Autodesk Inventor part; units mm, degrees
ref_plane "YZ Plane" through (0, 0, 0) normal (1, 0, 0) x (0, 1, 0)
ref_plane "XZ Plane" through (0, 0, 0) normal (0, 1, 0) x (-1, 0, 0)
ref_plane "XY Plane" through (0, 0, 0) normal (0, 0, 1) x (1, 0, 0)
sketch "Sketch1" plane through (0, 0, 0) normal (0, 1, 0) x (-1, 0, 0)
  line L0 (0, 0) -> (19.05, 0)
  line L1 (19.05, 0) -> (19.05, 44.45)
  line L2 (0, 19.05) -> (0, 0)
  circle A0 centre (9.525, 9.525) radius 6.35
  arc A1 (-166.7131, 44.45) -> (-166.7131, 19.05) centre (-215.9, 31.75) ccw
  line L3 (19.05, 44.45) -> (-41.3006, 44.45)
  line L4 (-139.6744, 44.45) -> (-166.7131, 44.45)
  line L5 (-166.7131, 19.05) -> (-139.6744, 19.05)
  line L6 (-41.3006, 19.05) -> (0, 19.05)
  arc A2 (-41.3006, 44.45) -> (-139.6744, 44.45) centre (-90.4875, 31.75) ccw
  arc A3 (-139.6744, 19.05) -> (-41.3006, 19.05) centre (-90.4875, 31.75) ccw
  dimension "d0" = 19.05
  dimension "d2" = 12.7
  dimension "d5" = 44.45
extrude "Extrusion1" add sketch "Sketch1" along normal blind 25.4
properties part number "wheels"
Read the model definition and answer for the solid it produces. Units are mm, in the model's axes. A direction names the side the tool comes from. Coordinates: 2 decimals unless noted, no trailing zeros. Write each loop counter-clockwise with the first axis right and the second up, starting at its lowest first coordinate (ties: lowest second). Pieces come first, ordered by that corner, then holes. Notation, with made-up numbers: (88, 59.5) - (136, 59.5) arc R15 cw to (136, 65.5) - close; hole circle Ø5 at (27, -32). An arc over 180 degrees is marked (long way). Answer as a JSON object with one key per item and string values. Group by question number.
1. A cutting plane is placed at D-D (z = 69.5). Determine the outline of the cut face in (x, y).
2. A cutting plane is placed at C-C (z = 13). Determine the outline of the cut face in (x, y), plus the area to 3 significant figures.
3. Which of the six approach directions +Z, -Z, +X, -X, +Y, -Y give full straight-line access (tool end or side, diameter ignored) to faces 1 (the flat face through (153, 13, 19.05)), 2 (the flat face through (153, 13, 44.45)), 3 (the flat face through (-9, 13, 0))?
4. Each of these flat-tipped pins is pushed along its axis until it touches: P1, Ø1.5, axis at y = 21, z = 69, coming from the +X side; P2, Ø15, axis at x = -7.5, y = 9.5, coming from the -Z side; P3, Ø1.5, axis at x = 86, y = 19.5, coming from the -Z side. Where does it stop, or does it pass through?
5. A cutting plane is placed at A-A (z = 52). Determine the outline of the cut face in (x, y).
6. The mould has two halves that part along X. Classify faces 4 (the flat face through (126, 25.4, 32)), 5 (the flat face through (-19.05, 13, 22)), 6 (the cylindrical face through (91.42, 12.52, 82.54)): +X half, -X half, draft (parallel to the pull), parting line (faces both ways), or undercut.
7. Consider L1, parallel to X at y = 11, z = 5; L2, parallel to X at y = 19, z = 0.5; L3, parallel to X at y = 8.25, z = 19. Determine where each line is inside the solid, lowest interval first. Write a range as [from, to].
Worked out:
{
 "1": {"outline": "(56.49, 0) - (124.48, 0) - (124.48, 25.4) - (56.49, 25.4) - close; (181.91, 0) - (249.89, 0) - (249.89, 25.4) - (181.91, 25.4) - close"},
 "2": {"outline": "(-19.05, 0) - (-14.84, 0) - (-14.84, 25.4) - (-19.05, 25.4) - close; (-4.21, 0) - (0, 0) - (0, 25.4) - (-4.21, 25.4) - close; (43.27, 0) - (137.7, 0) - (137.7, 25.4) - (43.27, 25.4) - close; (168.69, 0) - (263.11, 0) - (263.11, 25.4) - (168.69, 25.4) - close", "area": "5,010 mm²"},
 "3": {"face 1": "-Z, +Y, -Y", "face 2": "+Z, +Y, -Y", "face 3": "-Z, -X, +Y, -Y"},
 "4": {"P1": "stops at x = 251.23", "P2": "stops at z = 0", "P3": "stops at z = -18.91"},
 "5": {"outline": "(43.9, 0) - (137.08, 0) - (137.08, 25.4) - (43.9, 25.4) - close; (169.31, 0) - (262.49, 0) - (262.49, 25.4) - (169.31, 25.4) - close"},
 "6": {"face 4": "draft", "face 5": "-X half", "face 6": "undercut"},
 "7": {"L1": "x = [-19.05, -13.98], [-5.07, 0], [47.3, 133.67], [172.71, 259.09]", "L2": "x = [-19.05, 0], [50.44, 130.54], [175.85, 255.95]", "L3": "x = [-19.05, 0], [41.31, 139.66], [166.73, 265.07]"}
}
